```python
from build123d import *

# Parameters (mm, degrees)
F1_DEPTH = 5
F2_SIZE  = 0.1
F3_W     = 0.5
F3_H     = 0.4


with BuildPart() as f1:
    # F0 (on Top) → F1 (new body)
    with BuildSketch(Plane.XY):
        with BuildLine():
            Line((-2.291288, -1), (2.291288, -1))
            ThreePointArc((2.291288, -1), (0, 2.5), (-2.291288, -1))
        make_face()
    extrude(amount=F1_DEPTH)

    # F2
    f2_edges = [f1.edges().sort_by_distance(p)[0] for p in [
        (0, -1, 5),
        (0, 2.5, 5),
    ]]
    chamfer(f2_edges, length=F2_SIZE)

    # F5: sweep along a path in F4
    with BuildLine(Plane.XZ) as f5_path:
        Line((-1.27, 0), (-1.27, -1.792893))
        ThreePointArc((-1.27, -1.792893), (-1.30806, -1.984235), (-1.416447, -2.146447))
        Line((-1.416447, -2.146447), (-2.393553, -3.123553))
        ThreePointArc((-2.393553, -3.123553), (-2.50194, -3.285765), (-2.54, -3.477107))
        Line((-2.54, -3.477107), (-2.54, -6.77))
    # F3 (on face) → F5 (sweep)
    with BuildSketch(Plane(origin=(0, 0, 0), x_dir=(1, 0, 0), z_dir=(0, 0, -1))):
        with Locations((-1.27, 0)):
            Rectangle(F3_W, F3_H)
    sweep(path=f5_path.line)

    # F6: sweep along a path in F4
    with BuildLine(Plane.XZ) as f6_path:
        Line((0, 0), (0, -6.77))
    # F3 (on face) → F6 (sweep)
    with BuildSketch(Plane(origin=(0, 0, 0), x_dir=(1, 0, 0), z_dir=(0, 0, -1))):
        Rectangle(F3_W, F3_H)
    sweep(path=f6_path.line)

    # F7: sweep along a path in F4
    with BuildLine(Plane.XZ) as f7_path:
        Line((1.27, 0), (1.27, -1.792893))
        ThreePointArc((1.27, -1.792893), (1.30806, -1.984235), (1.416447, -2.146447))
        Line((1.416447, -2.146447), (2.393553, -3.123553))
        ThreePointArc((2.393553, -3.123553), (2.50194, -3.285765), (2.54, -3.477107))
        Line((2.54, -3.477107), (2.54, -6.77))
    # F3 (on face) → F7 (sweep)
    with BuildSketch(Plane(origin=(0, 0, 0), x_dir=(1, 0, 0), z_dir=(0, 0, -1))):
        with Locations((1.27, 0)):
            Rectangle(F3_W, F3_H)
    sweep(path=f7_path.line)


solid = f1.part
```
Read the model definition and answer for the solid it produces. Units are mm, in the model's axes. A direction names the side the tool comes from. Give positions to 0.01 mm unless a question says otherwise; leave off trailing zeros. Loops run counter-clockwise (first coordinate to the right, second up) from the corner with the lowest first, then second, coordinate; pieces in that order, holes last.
Item 1: Each of these flat-tipped pins is pushed along its axis until it touches: pin 1 Ø1.8 at (x, y) = (0, 1.5) entering from -Z; pin 2 Ø0.9 at (x, z) = (-2, -4) entering from +Y; pin 3 Ø1.4 at (x, z) = (-1.5, -2.5) entering from -Y. Where does it stop, or does it pass through?
Item 2: The part is cut by section A-A (z = -4). Write down the section's boundary in (x, y), and give its area (3 significant figures).
Item 3: For faces 1 (the flat face through (-2.29, -0.2, -3.15)), 2 (the flat face through (-1.735, 0.003, -2.819)), 3 (the flat face through (2.089, 0.003, -2.465)), determine the directions among +Z, -Z, +X, -X, +Y, -Y from which every point of the face is accessible in a straight line to the end or side of a thin tool.
Item 4: Find the intervals of material crossed by line 1 along X through (y, z) = (-0.1, -5.25); line 2 along Z through (x, y) = (0.05, 1.6); line 3 along X through (y, z) = (0.05, 1.75), in increasing order.
Item 5: The mould has two halves that part along Z. Classify faces 4 (the flat face through (0, 0, 5)), 5 (the flat face through (-2.089, -0.003, -2.465)), 6 (the flat face through (2.29, 0.2, -3.15)): released by +Z, released by -Z, zero draft, split by the parting line, or undercut.
Item 6: The part is cut by section B-B (x = 0). Write down the section's boundary in (y, z), and give its area (3 significant figures).
Item 7: The part is cut by section D-D (z = -2.5). Write down the section's boundary in (x, y).
Taken from the geometry:
1. pin 1: stops at z = 0
1. pin 2: stops at y = 0.2
1. pin 3: stops at y = -0.2
2. outline: (-2.79, -0.2) - (-2.29, -0.2) - (-2.29, 0.2) - (-2.79, 0.2) - close; (-0.25, -0.2) - (0.25, -0.2) - (0.25, 0.2) - (-0.25, 0.2) - close; (2.29, -0.2) - (2.79, -0.2) - (2.79, 0.2) - (2.29, 0.2) - close
2. area: 0.600 mm2
3. face 1: -Z, +X, -X, -Y
3. face 2: -Z, +Y, -Y
3. face 3: +X, +Y, -Y
4. line 1: x = -2.79 to -2.29, -0.25 to 0.25, 2.29 to 2.79
4. line 2: z = 0 to 5
4. line 3: x = -2.5 to 2.5
5. face 4: released by +Z
5. face 5: undercut
5. face 6: zero draft
6. outline: (-1, 0) - (-0.2, 0) - (-0.2, -6.77) - (0.2, -6.77) - (0.2, 0) - (2.5, 0) - (2.5, 4.9) - (2.4, 5) - (-0.9, 5) - (-1, 4.9) - close
6. area: 20.2 mm2
7. outline: (-2.12, -0.2) - (-1.42, -0.2) - (-1.42, 0.2) - (-2.12, 0.2) - close; (-0.25, -0.2) - (0.25, -0.2) - (0.25, 0.2) - (-0.25, 0.2) - close; (1.42, -0.2) - (2.12, -0.2) - (2.12, 0.2) - (1.42, 0.2) - close
